Input: part model. Units: mm. Frame: model coordinates. A direction names the side the tool comes from. Coordinates: 2 decimals unless noted, no trailing zeros. Write each loop counter-clockwise with the first axis right and the second up, starting at its lowest first coordinate (ties: lowest second). Pieces come first, ordered by that corner, then holes. Notation, with made-up numbers: (58, 74) - (79, 74) arc R19 cw to (79, 108) - close; hole circle Ø7 at (-5.75, -10.5). An arc over 180 degrees is marked (long way). Put each result on its own line as item: value. Start each with the question number.
1. Cut plane C-C, the plane x = 6.25. Return loops of the section in (y, z), and give its area (3 significant figures).
2. Pull-direction query (Y, two-part tool) for faces 1 (the cylindrical face through (-7.83, 0.82, 9.54)), 2 (the flat face through (8.1, 0, 12.5)), 3 (the cylindrical face through (0.053, 7.874, 9.542)), 4 (the flat face through (13, -4.182, 6)); classes: released by +Y, released by -Y, zero draft, split by the parting line, or undercut.
3. Line query: line 1 (Y direction, x = 12.25, z = 6.75); line 2 (Y direction, x = 4.5, z = 6.75); line 3 (Y direction, x = 1.75, z = 11.75). Output: solid intervals per line, ascending.
4. Pin query (flat end, axial travel): pin 1 (1.6 mm diameter, centred on x = 12, z = 7, fed in from +Y); pin 2 (4 mm diameter, centred on x = 3.5, z = 10.5, fed in from -Y); pin 3 (1.5 mm diameter, centred on x = -4.5, y = 0, fed in from +Z); pin 4 (4.5 mm diameter, centred on x = 13.5, z = 5.5, fed in from -Y). Return the tip coordinate at first contact, or that it passes through.
5. Cut plane B-B, the plane z = 5. Return loops of the section in (x, y) (3 decimals).
6. Access query for faces 5 (the flat face through (5, -5, 0)), 6 (the flat face through (13, 3.318, 6)), 7 (the cylindrical face through (-6.83, 7.35, 9.54)). Directions: +Z, -Z, +X, -X, +Y, -Y. A direction counts if a zero-diameter tool reaches every point of the face in a straight line with its end or side. Return the directions, or none.
7. Cut plane D-D, the plane z = 11. Return loops of the section in (x, y).
8. Cut plane A-A, the plane x = 0. Return loops of the section in (y, z) (3 decimals), and give its area (3 significant figures).
from build123d import *

# Parameters (mm, degrees)
F0_R     = 10.668
F1_DEPTH = 12.5
F3_DEPTH = 6
F4_DEPTH = 12.5
F5_W     = 5.5
F5_H     = 7.5
F6_DEPTH = 12.5


with BuildPart() as f1:
    # F0 (on Top) → F1 (new body)
    with BuildSketch(Plane.XY):
        Circle(F0_R)
    extrude(amount=F1_DEPTH)

    # F2 (on face) → F3 (cut)
    with BuildSketch(Plane.XY.offset(12.5)):
        with BuildLine():
            ThreePointArc((7.4103049922, -2.6621900614), (7.7572101141, -1.3511355394), (7.874, 0))
            ThreePointArc((7.874, 0), (7.5870287926, 2.1063879275), (6.7470327404, 4.0592394854))
            ThreePointArc((6.7470327404, 4.0592394854), (5.3099885026, 3.5816895419), (3.9127477219, 4.1655288097))
            ThreePointArc((3.9127477219, 4.1655288097), (5.2451205053, 2.2693470172), (5.715, 0))
            ThreePointArc((5.715, 0), (5.4426248431, -1.7432899407), (4.6514620061, -3.3204105477))
            ThreePointArc((4.6514620061, -3.3204105477), (5.9076375819, -2.4747315537), (7.4103049922, -2.6621900614))
        make_face()
        with BuildLine():
            ThreePointArc((3.9127477219, 4.1655288097), (5.3099885026, 3.5816895419), (6.7470327404, 4.0592394854))
            ThreePointArc((6.7470327404, 4.0592394854), (5.3908968998, 5.7391729906), (3.6294620987, 6.9876234067))
            ThreePointArc((3.6294620987, 6.9876234067), (3.2426928667, 5.5235334018), (3.9127477219, 4.1655288097))
        make_face()
        with BuildLine():
            ThreePointArc((3.6294620987, 6.9876234067), (5.3908968998, 5.7391729906), (6.7470327404, 4.0592394854))
            ThreePointArc((6.7470327404, 4.0592394854), (7.3388674181, 4.8082101234), (7.5498968998, 5.7391729906))
            ThreePointArc((7.5498968998, 5.7391729906), (6.0460088233, 7.7963821116), (3.6294620987, 6.9876234067))
        make_face()
        with BuildLine():
            ThreePointArc((8.5676809877, -4.5747878637), (8.2558121722, -3.4570278774), (7.4103049922, -2.6621900614))
            ThreePointArc((7.4103049922, -2.6621900614), (6.4086809877, -4.5747878637), (4.9252388756, -6.1434434984))
            ThreePointArc((4.9252388756, -6.1434434984), (7.2626509755, -6.557719093), (8.5676809877, -4.5747878637))
        make_face()
        with BuildLine():
            ThreePointArc((4.9252388756, -6.1434434984), (6.4086809877, -4.5747878637), (7.4103049922, -2.6621900614))
            ThreePointArc((7.4103049922, -2.6621900614), (5.9076375819, -2.4747315537), (4.6514620061, -3.3204105477))
            ThreePointArc((4.6514620061, -3.3204105477), (4.2597626921, -4.7831893008), (4.9252388756, -6.1434434984))
        make_face()
        with BuildLine():
            ThreePointArc((3.9127477219, 4.1655288097), (3.2426928667, 5.5235334018), (3.6294620987, 6.9876234067))
            ThreePointArc((3.6294620987, 6.9876234067), (0, 7.874), (-3.6294620987, 6.9876234067))
            ThreePointArc((-3.6294620987, 6.9876234067), (-3.3336877788, 6.394284914), (-3.2318968998, 5.7391729906))
            ThreePointArc((-3.2318968998, 5.7391729906), (-3.4094069377, 4.8818641023), (-3.9127477844, 4.165528751))
            ThreePointArc((-3.9127477844, 4.165528751), (-4.29e-08, 5.715), (3.9127477219, 4.1655288097))
        make_face()
        with BuildLine():
            ThreePointArc((-4.9252388756, -6.1434434984), (0, -7.874), (4.9252388756, -6.1434434984))
            ThreePointArc((4.9252388756, -6.1434434984), (4.2597626921, -4.7831893008), (4.6514620061, -3.3204105477))
            ThreePointArc((4.6514620061, -3.3204105477), (6.6e-09, -5.715), (-4.6514619984, -3.3204105585))
            ThreePointArc((-4.6514619984, -3.3204105585), (-4.3525782668, -3.9162116714), (-4.2496809877, -4.5747878637))
            ThreePointArc((-4.2496809877, -4.5747878637), (-4.4257497584, -5.4287578515), (-4.9252388756, -6.1434434984))
        make_face()
        with BuildLine():
            ThreePointArc((-3.2318968998, 5.7391729906), (-3.3336877788, 6.394284914), (-3.6294620987, 6.9876234067))
            ThreePointArc((-3.6294620987, 6.9876234067), (-5.3908968998, 5.7391729906), (-6.7470327404, 4.0592394854))
            ThreePointArc((-6.7470327404, 4.0592394854), (-5.3099885454, 3.5816895403), (-3.9127477844, 4.165528751))
            ThreePointArc((-3.9127477844, 4.165528751), (-3.4094069377, 4.8818641023), (-3.2318968998, 5.7391729906))
        make_face()
        with BuildLine():
            ThreePointArc((-6.7470327404, 4.0592394854), (-5.3908968998, 5.7391729906), (-3.6294620987, 6.9876234067))
            ThreePointArc((-3.6294620987, 6.9876234067), (-6.8690460498, 7.3128171977), (-6.7470327404, 4.0592394854))
        make_face()
        with BuildLine():
            ThreePointArc((-4.6514619984, -3.3204105585), (-5.6873758569, 0.5612315586), (-3.9127477844, 4.165528751))
            ThreePointArc((-3.9127477844, 4.165528751), (-5.3099885454, 3.5816895403), (-6.7470327404, 4.0592394854))
            ThreePointArc((-6.7470327404, 4.0592394854), (-7.8359400653, 0.7732524124), (-7.4103049922, -2.6621900614))
            ThreePointArc((-7.4103049922, -2.6621900614), (-5.9076375754, -2.4747315552), (-4.6514619984, -3.3204105585))
        make_face()
        with BuildLine():
            ThreePointArc((-7.4103049922, -2.6621900614), (-8.1658999682, -5.8291651812), (-4.9252388756, -6.1434434984))
            ThreePointArc((-4.9252388756, -6.1434434984), (-6.4086809877, -4.5747878637), (-7.4103049922, -2.6621900614))
        make_face()
        with BuildLine():
            ThreePointArc((-7.4103049922, -2.6621900614), (-6.4086809877, -4.5747878637), (-4.9252388756, -6.1434434984))
            ThreePointArc((-4.9252388756, -6.1434434984), (-4.4257497584, -5.4287578515), (-4.2496809877, -4.5747878637))
            ThreePointArc((-4.2496809877, -4.5747878637), (-4.3525782668, -3.9162116714), (-4.6514619984, -3.3204105585))
            ThreePointArc((-4.6514619984, -3.3204105585), (-5.9076375754, -2.4747315552), (-7.4103049922, -2.6621900614))
        make_face()
    extrude(amount=-F3_DEPTH, mode=Mode.SUBTRACT)

    # F4 (cut): a face of the model
    f4_faces = [f1.faces().sort_by_distance(p)[0] for p in [
        (0, 0, 12.5),
    ]]
    extrude(f4_faces, amount=-F4_DEPTH, mode=Mode.SUBTRACT)

    # F5 (on Top) → F6 (join)
    with BuildSketch(Plane.XY):
        with Locations((12.6280929255, -0.4317085259)):
            Rectangle(F5_W, F5_H)
    extrude(amount=F6_DEPTH)


solid = f1.part
Report:
1. outline: (-8.65, 0) - (8.65, 0) - (8.65, 12.5) - (7.72, 12.5) - (7.72, 6.5) - (-6.73, 6.5) - (-6.73, 12.5) - (-8.65, 12.5) - close
1. area: 129 mm^2
2. face 1: undercut
2. face 2: zero draft
2. face 3: undercut
2. face 4: released by -Y
3. line 1: y = -4.18 to 3.32
3. line 2: y = -9.67 to -6.46, 7.71 to 9.67
3. line 3: y = -10.52 to -7.68, 7.68 to 10.52
4. pin 1: stops at y = 3.32
4. pin 2: stops at y = -10.56
4. pin 3: passes through
4. pin 4: stops at y = -4.18
5. outline: (9.878, -4.182) - (15.378, -4.182) - (15.378, 3.318) - (10.139, 3.318) arc R10.668 ccw (long way) to (9.878, -4.029) - close; hole circle Ø11.43 at (0, 0)
6. face 5: -Z, +X, -X, +Y, -Y
6. face 6: +Z, -Z, +X, +Y
6. face 7: +Z
7. outline: (9.88, -4.18) - (15.38, -4.18) - (15.38, 3.32) - (10.14, 3.32) arc R10.67 ccw (long way) to (9.88, -4.03) - close; hole (-7.41, -2.66) arc R2.16 ccw (long way) to (-4.93, -6.14) arc R7.87 ccw to (4.93, -6.14) arc R2.16 ccw (long way) to (7.41, -2.66) arc R7.87 ccw to (6.75, 4.06) arc R2.16 ccw (long way) to (3.63, 6.99) arc R7.87 ccw to (-3.63, 6.99) arc R2.16 ccw (long way) to (-6.75, 4.06) arc R7.87 ccw to start
8. outline: (-10.668, 0) - (-5.715, 0) - (-5.715, 6.5) - (-7.874, 6.5) - (-7.874, 12.5) - (-10.668, 12.5) - close; (5.715, 0) - (10.668, 0) - (10.668, 12.5) - (7.874, 12.5) - (7.874, 6.5) - (5.715, 6.5) - close
8. area: 97.9 mm^2
